```python
from build123d import *

# Parameters (mm, degrees)
BOSS_EXTRUDE1_DEPTH = 26
SHELL1_T            = -2
SKETCH3_W           = 5
SKETCH3_H           = 15
CUT_EXTRUDE1_DEPTH  = 5
SKETCH4_R           = 1.5
CUT_EXTRUDE2_DEPTH  = 10
BOSS_EXTRUDE2_DEPTH = 3
SKETCH7_R           = 1.397
CUT_EXTRUDE3_DEPTH  = 5
SKETCH8_R           = 1.397
CUT_EXTRUDE4_DEPTH  = 5


with BuildPart() as part:
    # Sketch1 → Boss-Extrude1 (new body)
    with BuildSketch(Plane(origin=(0, 0, 0), x_dir=(1, 0, 0), z_dir=(0, 1, 0))):
        with BuildLine():
            Line((6.305887047, 78.84802453), (27.694112953, 78.84802453))
            ThreePointArc((27.694112953, 78.84802453), (30.374796425, 77.816851929), (31.673356222, 75.254992592))
            Line((31.673356222, 75.254992592), (36, 32.950031211))
            Line((36, 32.950031211), (36, -0.049968789))
            Line((36, -0.049968789), (35.092510916, -18.199750468))
            ThreePointArc((35.092510916, -18.199750468), (33.854401824, -20.898189251), (31.097501561, -22))
            Line((31.097501561, -22), (2.902498439, -22))
            ThreePointArc((2.902498439, -22), (0.145598176, -20.898189251), (-1.092510916, -18.199750468))
            Line((-1.092510916, -18.199750468), (-2, -0.049968789))
            Line((-2, -0.049968789), (-2, 32.950031211))
            Line((-2, 32.950031211), (2.326643778, 75.254992592))
            ThreePointArc((2.326643778, 75.254992592), (3.625203575, 77.816851929), (6.305887047, 78.84802453))
        make_face()
    extrude(amount=BOSS_EXTRUDE1_DEPTH)

    # Shell1
    shell1_openings = [part.faces().sort_by_distance(p)[0] for p in [
        (17, 0, -26.610641327),
    ]]
    offset(amount=SHELL1_T, openings=shell1_openings, kind=Kind.INTERSECTION)

    # Sketch3 → Cut-Extrude1 (cut)
    with BuildSketch(Plane.XY.offset(22)):
        with Locations((25.508858148, 7.5)):
            Rectangle(SKETCH3_W, SKETCH3_H)
    extrude(amount=-CUT_EXTRUDE1_DEPTH, mode=Mode.SUBTRACT)

    # Sketch4 → Cut-Extrude2 (cut)
    with BuildSketch(Plane.XZ.offset(-24)):
        with Locations(Location((17, -10, 0), (0, 0, 270))):
            Circle(SKETCH4_R)
        with Locations(Location((17, -32, 0), (0, 0, 270))):
            Circle(SKETCH4_R)
    extrude(amount=-CUT_EXTRUDE2_DEPTH, mode=Mode.SUBTRACT)

    # Sketch5 → Boss-Extrude2 (add)
    with BuildSketch(Plane.XZ):
        with BuildLine():
            Line((30.522727273, -66.84802453), (3.477272727, -66.84802453))
            Line((3.477272727, -66.84802453), (4.316265412, -75.051508561))
            ThreePointArc((4.316265412, -75.051508561), (4.965545311, -76.332438229), (6.305887047, -76.84802453))
            Line((6.305887047, -76.84802453), (27.694112953, -76.84802453))
            ThreePointArc((27.694112953, -76.84802453), (29.034454689, -76.332438229), (29.683734588, -75.051508561))
            Line((29.683734588, -75.051508561), (30.522727273, -66.84802453))
        make_face()
    extrude(amount=-BOSS_EXTRUDE2_DEPTH)

    # Sketch7 → Cut-Extrude3 (cut)
    with BuildSketch(Plane.XZ):
        with Locations(Location((24.335511696, -71.84802453, 0), (0, 0, 270))):
            Circle(SKETCH7_R)
    extrude(amount=-CUT_EXTRUDE3_DEPTH, mode=Mode.SUBTRACT)

    # Sketch8 → Cut-Extrude4 (cut)
    with BuildSketch(Plane.XZ):
        with Locations(Location((9.336175071, -71.84802453, 0), (0, 0, 270))):
            Circle(SKETCH8_R)
    extrude(amount=-CUT_EXTRUDE4_DEPTH, mode=Mode.SUBTRACT)


solid = part.part
```
Geometry check sheet. Reference: the model listing, model coordinates, mm. A direction names the side the tool comes from. Give positions to 0.01 mm unless a question says otherwise; leave off trailing zeros. Loops run counter-clockwise (first coordinate to the right, second up) from the corner with the lowest first, then second, coordinate; pieces in that order, holes last. Notation, with made-up numbers: M 64,80 L 120,80 A33 cw 120,118 Z; hole C 51,58.25 d9. An arc over 180 degrees is marked long. Answer as CSV lines item,"result".
Item 1: Release check for a two-part mould opening along Y. For faces 4 (the flat face through (31.81, 11.83, -54.25)), 5 (the flat face through (35.553, 12.818, 8.998)) record: pulls with the +Y half, pulls with the -Y half, needs draft (parallel to the pull), parting line crosses it, or undercut.
Values:
face 4,"undercut"
face 5,"needs draft"
Item 2: Material ranges on line 1 (X direction, y = 9, z = -9); line 2 (Z direction, x = 9, y = 20.5); line 3 (Y direction, x = 17, z = -67.5), recorded low to high.
Values:
line 1,"x = -2 to 0, 34 to 36"
line 2,"z = -78.85 to -76.85, 20 to 22"
line 3,"y = 0 to 3, 24 to 26"
Item 3: Cross-section at B-B on z = -10. Record the cut outline in (x, y), and give its area (3 significant figures).
Values:
outline,"M -2,0 L 0,0 L 0,24 L 15.5,24 L 15.5,26 L -2,26 Z; M 18.5,24 L 34,24 L 34,0 L 36,0 L 36,26 L 18.5,26 Z"
area,"166 mm²"
Item 4: Cross-section at A-A on x = 17. Record the cut outline in (y, z), and give its area (3 significant figures).
Values:
outline,"M 0,-78.85 L 26,-78.85 L 26,-33.5 L 24,-33.5 L 24,-76.85 L 3,-76.85 L 3,-66.85 L 0,-66.85 Z; M 0,20 L 24,20 L 24,-8.5 L 26,-8.5 L 26,22 L 0,22 Z; M 24,-30.5 L 26,-30.5 L 26,-11.5 L 24,-11.5 Z"
area,"316 mm²"
Item 5: Access from +Z, -Z, +X, -X, +Y, -Y to the whole of each face (thin tool, end or side, straight path). Record for faces 1 (the flat face through (34, 12, -17)), 2 (the flat face through (23.009, 7, 21)), 3 (the cylindrical face through (29.019, 13.353, -76.346)).
Values:
face 1,"-Y"
face 2,"+Z, -Y"
face 3,"none"
Item 6: Cross-section at D-D on y = 4.75. Record the cut outline in (x, z) (1 decimal), and give its area (3 significant figures).
Values:
outline,"M -2,-33 L 2.3,-75.3 A4 ccw 6.3,-78.8 L 27.7,-78.8 A4 ccw 31.7,-75.3 L 36,-33 L 36,0 L 35.1,18.2 A4 ccw 31.1,22 L 28,22 L 28,20 L 31.1,20 A2 cw 33.1,18.1 L 34,0 L 34,-32.8 L 29.7,-75.1 A2 cw 27.7,-76.8 L 6.3,-76.8 A2 cw 4.3,-75.1 L 0,-32.8 L 0,0 L 0.9,18.1 A2 cw 2.9,20 L 23,20 L 23,22 L 2.9,22 A4 ccw -1.1,18.2 L -2,0 Z"
area,"499 mm²"
Item 7: Cross-section at C-C on y = 20.5. Record the cut outline in (x, z) (1 decimal), and give its area (3 significant figures).
Values:
outline,"M -2,-33 L 2.3,-75.3 A4 ccw 6.3,-78.8 L 27.7,-78.8 A4 ccw 31.7,-75.3 L 36,-33 L 36,0 L 35.1,18.2 A4 ccw 31.1,22 L 2.9,22 A4 ccw -1.1,18.2 L -2,0 Z; hole M 0,-32.8 L 4.3,-75.1 A2 ccw 6.3,-76.8 L 27.7,-76.8 A2 ccw 29.7,-75.1 L 34,-32.8 L 34,0 L 33.1,18.1 A2 ccw 31.1,20 L 2.9,20 A2 ccw 0.9,18.1 L 0,0 Z"
area,"509 mm²"
Item 8: Depth check by flat-ended pin: P1, Ø1.6, axis at y = 6.5, z = 21, coming from the +X side; P2, Ø2.5, axis at x = 17, z = -10, coming from the +Y side; P3, Ø0.6, axis at y = 7.5, z = 20.5, coming from the -X side; P4, Ø10, axis at y = 15.5, z = -42.5, coming from the +X side. Enter the tip coordinate at first touch or a pass-through.
Values:
P1,"stops at x = 34.44"
P2,"passes through"
P3,"stops at x = -0.44"
P4,"stops at x = 35.53"
